Verification items for this drawing (mm, ordinates from the low corner). Coordinates: 2 decimals unless noted, no trailing zeros. Write each loop counter-clockwise with the first axis right and the second up, starting at its lowest first coordinate (ties: lowest second). Pieces come first, ordered by that corner, then holes.
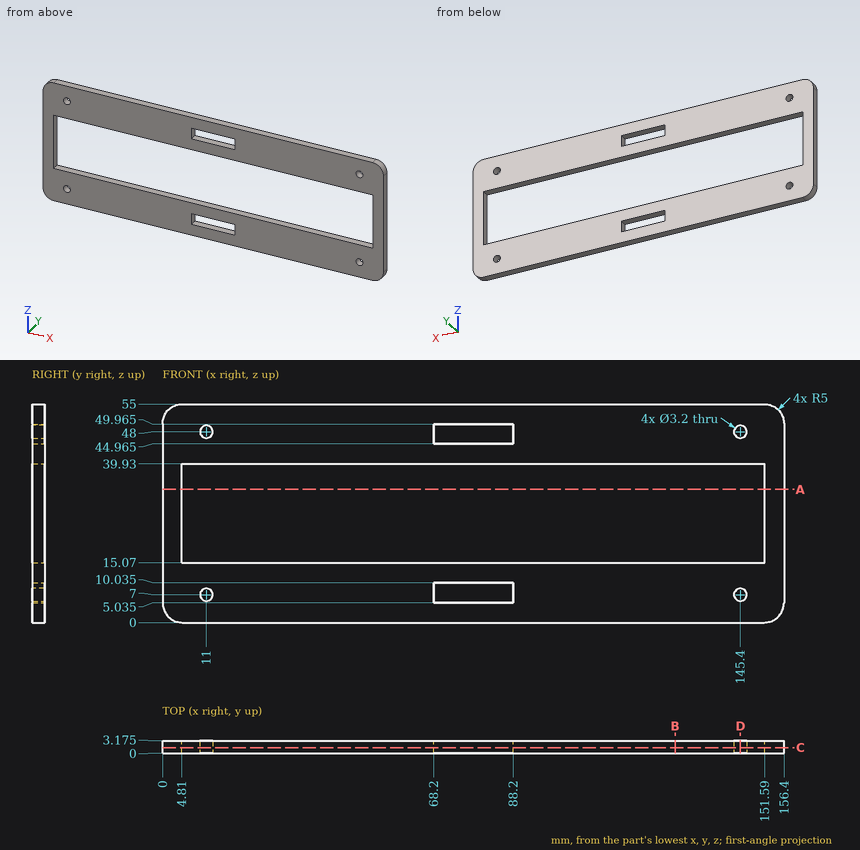
1. Sectioned sample at C-C, the plane y = 1.4. Record the boundary of the cut face in (x, z) (3 decimals).
Computed values:
outline: (0, 5) arc R5 ccw to (5, 0) - (151.4, 0) arc R5 ccw to (156.4, 5) - (156.4, 50) arc R5 ccw to (151.4, 55) - (5, 55) arc R5 ccw to (0, 50) - close; hole (4.81, 15.07) - (151.59, 15.07) - (151.59, 39.93) - (4.81, 39.93) - close; hole circle Ø3.2 at (11, 7); hole circle Ø3.2 at (11, 48); hole (68.2, 5.035) - (88.2, 5.035) - (88.2, 10.035) - (68.2, 10.035) - close; hole (68.2, 44.965) - (88.2, 44.965) - (88.2, 49.965) - (68.2, 49.965) - close; hole circle Ø3.2 at (145.4, 7); hole circle Ø3.2 at (145.4, 48)
2. Sectioned sample at A-A, the plane z = 33.5. Record the boundary of the cut face in (x, y) (3 decimals).
Computed values:
outline: (0, 0) - (4.81, 0) - (4.81, 3.175) - (0, 3.175) - close; (151.59, 0) - (156.4, 0) - (156.4, 3.175) - (151.59, 3.175) - close
3. Sectioned sample at D-D, the plane x = 145.4. Record the boundary of the cut face in (y, z) (3 decimals), and give its area (3 significant figures).
Computed values:
outline: (0, 0) - (3.175, 0) - (3.175, 5.4) - (0, 5.4) - close; (0, 8.6) - (3.175, 8.6) - (3.175, 15.07) - (0, 15.07) - close; (0, 39.93) - (3.175, 39.93) - (3.175, 46.4) - (0, 46.4) - close; (0, 49.6) - (3.175, 49.6) - (3.175, 55) - (0, 55) - close
area: 75.4 mm2
4. Thickness scan on line 1 along Z through (x, y) = (145.4, 1.3); line 2 along X through (y, z) = (1.65, 7); line 3 along Z through (x, y) = (83, 2.95) (3 decimals). Record the ranges inside material, lowest first.
Computed values:
line 1: z = 0 to 5.4, 8.6 to 15.07, 39.93 to 46.4, 49.6 to 55
line 2: x = 0 to 9.4, 12.6 to 68.2, 88.2 to 143.8, 147 to 156.4
line 3: z = 0 to 5.035, 10.035 to 15.07, 39.93 to 44.965, 49.965 to 55
5. Sectioned sample at B-B, the plane x = 129. Record the boundary of the cut face in (y, z) (3 decimals), and give its area (3 significant figures).
Computed values:
outline: (0, 0) - (3.175, 0) - (3.175, 15.07) - (0, 15.07) - close; (0, 39.93) - (3.175, 39.93) - (3.175, 55) - (0, 55) - close
area: 95.7 mm2
6. Gauge pin test, flat end, axial feed: pin 1 Ø1.9 at (x, z) = (11, 7) entering from -Y. Record the tip position at first contact, or that the pin passes through.
Computed values:
pin 1: passes through
